```python
from build123d import *

# Parameters (mm, degrees)
F1_DEPTH = 1150
F2_R     = 2
F4_DEPTH = 40.001


with BuildPart() as f1:
    # F0 (on Front) → F1 (new body)
    with BuildSketch(Plane.XZ):
        Polygon((0, 40), (0, 0), (32.190853, 0), (50, 40), align=None)
    extrude(amount=F1_DEPTH)

    # F2
    f2_edges = [f1.edges().sort_by_distance(p)[0] for p in [
        (50, -575, 40),
    ]]
    fillet(f2_edges, radius=F2_R)

    # F3 (on face) → F4 (cut, through all)
    with BuildSketch(Plane.XY.offset(40)):
        Polygon((46.92027, -1103.07973), (0, -1150), (46.92027, -1150), align=None)
        Polygon((53.244177, -1096.755823), (46.92027, -1103.07973), (46.92027, -1150), (53.244177, -1150), align=None)
    extrude(amount=-F4_DEPTH, mode=Mode.SUBTRACT)


solid = f1.part
```
The model under review builds one solid part; all positions refer to its coordinate system, in mm. Round coordinates to 2 decimals unless told otherwise and drop trailing zeros. Loops run counter-clockwise (first coordinate to the right, second up) from the corner with the lowest first, then second, coordinate; pieces in that order, holes last. Notation, with made-up numbers: M -13.75,33.5 L -2.75,33.5 A28 ccw -2.75,68.5 Z; hole C 49.25,-18 d3. An arc over 180 degrees is marked long. Answer as a JSON object with one key per item and string values.
(1) Clearance check with flat-ended pins moving along their axes: P1, Ø8, axis at y = -673, z = 22, coming from the +X side; P2, Ø6, axis at x = 29, z = 29, coming from the -Y side; P3, Ø6, axis at y = -558.5, z = 5.5, coming from the +X side. State where each tip first meets the part, or that it passes through.
Resolved:
{"P1": "x = 43.77", "P2": "y = -1124", "P3": "x = 35.98"}
(2) Take a section at A-A on y = -756. Give the boundary of the cut face in (x, z), and give its area (3 significant figures).
Resolved:
{"outline": "M 0,0 L 32.19,0 L 48.75,37.19 A2 ccw 46.92,40 L 0,40 Z", "area": "1,640 mm²"}
(3) Take a section at B-B on x = 21. Give the boundary of the cut face in (y, z).
Resolved:
{"outline": "M -1129,0 L 0,0 L 0,40 L -1129,40 Z"}
(4) To check wall thickness, follow line 1 along X through (y, z) = (-782, 11); line 2 along Z through (x, y) = (46.5, -954.5); line 3 along Y through (x, z) = (25, 16). State the ranges of each line that lie inside material, in increasing order.
Resolved:
{"line 1": "0 to 37.09", "line 2": "32.14 to 40", "line 3": "-1125 to 0"}
(5) Take a section at C-C on z = 27.5. Give the boundary of the cut face in (x, y), and give its area (3 significant figures).
Resolved:
{"outline": "M 0,-1150 L 44.43,-1105.57 L 44.43,0 L 0,0 Z", "area": "50,100 mm²"}
